from build123d import *

# Parameters (mm, degrees)
SKETCH005_W             = 58
SKETCH005_H             = 20
SKETCH005_R             = 2.75
PAD004_DEPTH            = 8
SKETCH006_R             = 2.25
PAD005_DEPTH            = 4
POCKET005_DEPTH         = 4
SKETCH011_W             = 15
SKETCH011_H             = 2.666667
POCKET007_DEPTH         = 20
SKETCH012_W             = 18
SKETCH012_H             = 3
POCKET008_DEPTH         = 8
FILLET_R                = 0.5
POCKET009_DEPTH         = 20
BODY002_PLACEMENT_ANGLE = 180


with BuildPart() as part:
    # Sketch005 → Pad004 (new body)
    with BuildSketch(Plane.XZ):
        Rectangle(SKETCH005_W, SKETCH005_H)
        Circle(SKETCH005_R, mode=Mode.SUBTRACT)
    extrude(amount=PAD004_DEPTH)

    # Sketch006 (on Face4 of Pad004) → Pad005 (join)
    with BuildSketch(Plane(origin=(-29, 0, 0), x_dir=(0, 0, -1), z_dir=(-1, 0, 0))):
        with BuildLine():
            Line((-10, 0), (10, 0))
            Line((10, 0), (10, 45.5))
            ThreePointArc((10, 45.5), (0, 55.5), (-10, 45.5))
            Line((-10, 45.5), (-10, 0))
        make_face()
        with Locations((0, 50)):
            Circle(SKETCH006_R, mode=Mode.SUBTRACT)
    pad005 = extrude(amount=PAD005_DEPTH)

    # Mirrored003: Pad005 across YZ
    add(pad005.mirror(Plane.YZ))

    # Sketch007 (on Face5 of Mirrored003) → Pocket005 (cut)
    with BuildSketch(Plane.XZ.offset(8)):
        Polygon((4.113621, 2.375), (0, 4.75), (-4.113621, 2.375), (-4.113621, -2.375), (0, -4.75), (4.113621, -2.375), align=None)
    extrude(amount=-POCKET005_DEPTH, mode=Mode.SUBTRACT)

    # Sketch011 (on Face14 of Pocket005) → Pocket007 (cut)
    with BuildSketch(Plane(origin=(0, 0, 10), x_dir=(-1, 0, 0), z_dir=(0, 0, 1))):
        with Locations((-19.5, 4.333334)):
            Rectangle(SKETCH011_W, SKETCH011_H)
    pocket007 = extrude(amount=-POCKET007_DEPTH, mode=Mode.SUBTRACT)

    # Mirrored004: Pocket007 across YZ
    add(pocket007.mirror(Plane.YZ), mode=Mode.SUBTRACT)

    # Sketch012 (on Face3 of Mirrored004) → Pocket008 (cut)
    with BuildSketch(Plane(origin=(0, 0, 0), x_dir=(1, 0, 0), z_dir=(0, 1, 0))):
        with Locations((0, 8.5)):
            Rectangle(SKETCH012_W, SKETCH012_H)
    extrude(amount=-POCKET008_DEPTH, mode=Mode.SUBTRACT)

    # Fillet
    fillet_edges = [part.edges().sort_by_distance(p)[0] for p in [
        (0, -8, -7),
        (9, -8, -8.5),
        (-9, -8, -8.5),
    ]]
    fillet(fillet_edges, radius=FILLET_R)

    # Sketch013 (on Face35 of Fillet) → Pocket009 (cut)
    with BuildSketch(Plane(origin=(0, 0, 10), x_dir=(-1, 0, 0), z_dir=(0, 0, 1))):
        Polygon((-29, 0), (-32.156707, 2.74), (-33, 4), (-33, 0), align=None)
    extrude(amount=-POCKET009_DEPTH, mode=Mode.SUBTRACT)


with BuildPart() as part_1:
    # Body002 placement: moved
    add(part.part.moved(Location((-14.3, -30, 19.9))).rotate(Axis((-14.3, -30, 19.9), (1, 0, 0)), BODY002_PLACEMENT_ANGLE))


solid = part_1.part
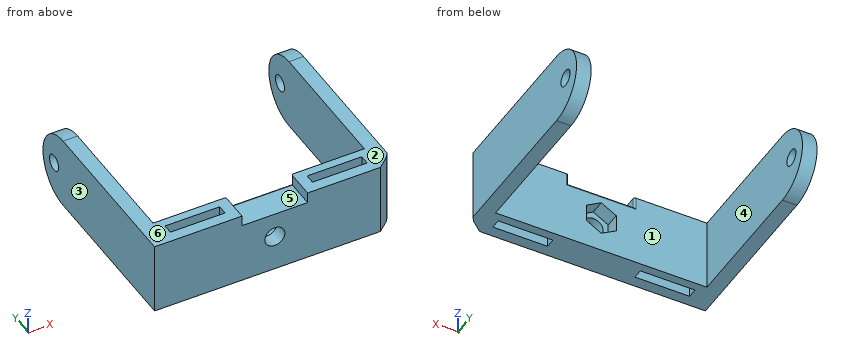
Here's how the part is built. I have some questions about the finished solid (model axes, mm). Face numbers are marked on the shaded views. A direction names the side the tool comes from. Give positions to 0.01 mm unless a question says otherwise; leave off trailing zeros. Order: outer loops, then holes, each group sorted by start corner. A loop starts at its lowest first (then second) coordinate and runs counter-clockwise, first axis right, second up. Notation, with made-up numbers: M 75,-1.75 L 105,-1.75 A22 ccw 105,6.25 Z; hole C 37.25,17 d9. An arc over 180 degrees is marked long. Answer as a JSON object with one key per item and string values. Group by question number.
1) Suppose I cut it at B-B, the plane y = 9. Write out the boundary of the cut face in (x, z), plus the area to 3 significant figures.
2) Suppose I cut it at C-C, the plane x = 7. Write out the boundary of the cut face in (y, z).
3) Suppose I cut it at D-D, the plane z = 13.5. Write out the boundary of the cut face in (x, y), plus the area to 3 significant figures.
4) Please list where these lines run through material, in increasing order: L1, parallel to X at y = 15, z = 26.25; L2, parallel to X at y = -24, z = 22.25; L3, parallel to Z at x = -14.3, y = -28.4. Write a range as [from, to].
5) On a 3-axis mill with a long thin cutter (end or side, diameter ignored), from which of +Z, -Z, +X, -X, +Y, -Y can I reach the whole of each face in a straight line? I mean the marked faces 1 and 2. Say none if no direction works.
6) Suppose I cut it at A-A, the plane z = 19.9. Count the separate pieces of the cut face and the enclosed holes in it, plus the area to 3 significant figures.
7) We'd pull the mould along X, two halves only. Please class the marked faces 3, 4, 5 and 6: pulls with the +X half, pulls with the -X half, needs draft (parallel to the pull), parting line crosses it, or undercut.
8) I'm going to push a flat-ended pin straight in: pin 1 Ø1.5 at (y, z) = (-27.5, 28.5) entering from +X. Where does the tip first touch, or does it pass through?
Results found:
{
 "1": {"outline": "M -47.3,9.9 L -43.3,9.9 L -43.3,29.9 L -47.3,29.9 Z; M 14.7,9.9 L 18.7,9.9 L 18.7,29.9 L 14.7,29.9 Z", "area": "160 mm²"},
 "2": {"outline": "M -30,9.9 L -27,9.9 L -27,29.9 L -30,29.9 Z; M -24.33,9.9 L -22,9.9 L -22,29.9 L -24.33,29.9 Z"},
 "3": {"outline": "M -47.3,-30 L 14.7,-30 L 17.86,-27.26 L 18.7,-26 L 18.7,23.18 L 14.7,23.18 L 14.7,-22 L -43.3,-22 L -43.3,23.18 L -47.3,23.18 Z; hole M -41.3,-27 L -26.3,-27 L -26.3,-24.33 L -41.3,-24.33 Z; hole M -2.3,-27 L 12.7,-27 L 12.7,-24.33 L -2.3,-24.33 Z", "area": "802 mm²"},
 "4": {"L1": "[-47.3, -43.3], [14.7, 18.7]", "L2": "[-47.3, -18.41], [-10.19, 18.7]", "L3": "[9.9, 17.15], [22.65, 26.9]"},
 "5": {"face 1": "+Z, -Z, +Y", "face 2": "+Z, +X, -X, +Y, -Y"},
 "6": {"separate pieces": "4", "enclosed holes": "2", "area": "730 mm²"},
 "7": {"face 3": "pulls with the -X half", "face 4": "undercut", "face 5": "undercut", "face 6": "needs draft"},
 "8": {"pin 1": "x = 18.2"}
}
